Can you work these out from the drawing? Everything is in mm from the part's minimum corner. Coordinates: 2 decimals unless noted, no trailing zeros. Loops run counter-clockwise (first coordinate to the right, second up) from the corner with the lowest first, then second, coordinate; pieces in that order, holes last. Notation, with made-up numbers: (-13, 22.5) -> (-3, 22.5) arc R12 ccw to (-3, 41.5) -> close; hole circle Ø6 at (28.5, 11). An arc over 180 degrees is marked (long way). Use one line per item in the form item = value. Start each with the question number.
(1) Imagine slicing it at D-D (z = 6.5). List the corners of the cut face in (x, y) for me.
(2) I need wall thicknesses on line 1 (Y direction, x = 3.5, z = 1.4); line 2 (Z direction, x = 6, y = 3); line 3 (Z direction, x = 4.5, y = 3.75). Which ranges of each line are inside material? Lowest first, please. Write a range as [from, to].
(3) Imagine slicing it at C-C (z = 1.5). List the corners of the cut face in (x, y) for me, plus the area to 3 significant figures.
(4) Thinking about a two-plate mould opening in Y: for the marked faces 1, 2 and 3, which applies, released by +Y, released by -Y, zero draft, split by the parting line, or undercut?
(5) I'm going to push flat-ended pins straight in: pin 1 (4 mm diameter, centred on x = 3.5, y = 6, fed in from +Z); pin 2 (3 mm diameter, centred on x = 6, z = 9, fed in from -Y); pin 3 (1 mm diameter, centred on x = 3, y = 3.5, fed in from -Z); pin 4 (3 mm diameter, centred on x = 1, z = 6.5, fed in from +Y). Where does each tip first touch, or does it pass through?
(6) Imagine slicing it at A-A (y = 3.5). List the corners of the cut face in (x, z) for me, plus the area to 3 significant figures.
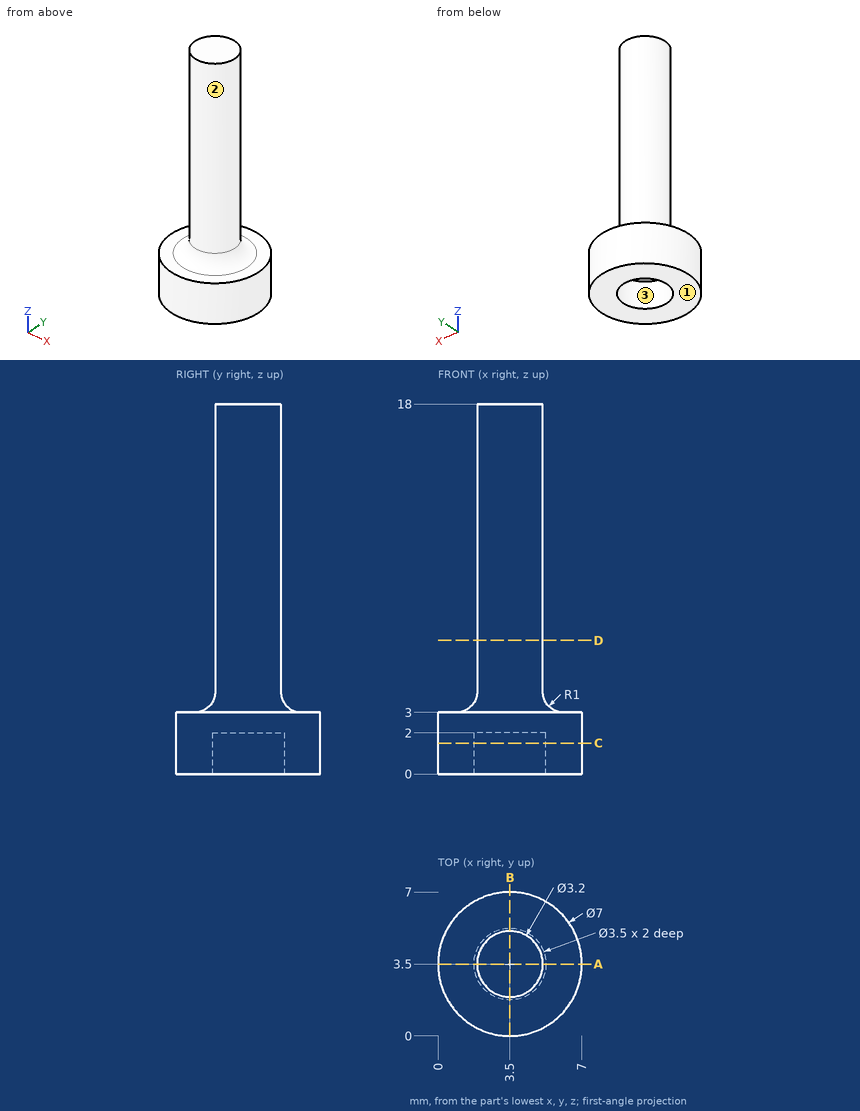
Worked out:
q1.outline = circle Ø3.2 at (3.5, 3.5)
q2.line_1 = [0, 1.75], [5.25, 7]
q2.line_2 = [0, 3]
q2.line_3 = [2, 18]
q3.outline = circle Ø7 at (3.5, 3.5); hole circle Ø3.5 at (3.5, 3.5)
q3.area = 28.9 mm2
q4.face_1 = zero draft
q4.face_2 = split by the parting line
q4.face_3 = undercut
q5.pin_1 = 18
q5.pin_2 = 2.25
q5.pin_3 = 2
q5.pin_4 = 4.75
q6.outline = (0, 0) -> (1.75, 0) -> (1.75, 2) -> (5.25, 2) -> (5.25, 0) -> (7, 0) -> (7, 3) -> (6.1, 3) arc R1 cw to (5.1, 4) -> (5.1, 18) -> (1.9, 18) -> (1.9, 4) arc R1 cw to (0.9, 3) -> (0, 3) -> close
q6.area = 62.4 mm2
